from build123d import *

# Parameters (mm, degrees)
SKETCH_1_R               = 40
SKETCH_2_R               = 33.35
SKETCH_3_R               = 2.2
CUT_EXTRUDE_1_DEPTH      = 57.789083608
SKETCH_4_R               = 4
CUT_EXTRUDE_2_DEPTH      = 3
OTHER_START              = -5
OTHER_1_OUTLINE_R        = 4
OTHER_1_OUTLINE_R_2      = 2.9
OTHER_1_OUTLINE_R_3      = 11
OTHER_1_OUTLINE_R_4      = 9
OTHER_1_DEPTH            = 1.5
CUT_EXTRUDE_START        = 27
SKETCH_5_R               = 11.2
SKETCH_5_R_2             = 4.2
CUT_EXTRUDE_3_DEPTH      = 1.5
SKETCH_7_R               = 2.2
EXTRUDE_1_DEPTH          = 5
HOLE_WIZARD_4_4_4_4_1_D  = 4.4
CUT_EXTRUDE_4_DEPTH      = 91.740732016
CUT_EXTRUDE_4_DEPTH_BACK = 91.740732016


# Read off the part's stored shape, not the designer's step: 型腔1
with BuildPart() as part:
    # 草图1 → 放样2 section 0
    with BuildSketch(Plane.XY):
        Circle(SKETCH_1_R)
    # 草图2 → 放样2 section 1
    with BuildSketch(Plane.XY.offset(-5)):
        Circle(SKETCH_2_R)
    loft()

    # 草图3 → 切除-拉伸1 (cut, through all)
    with BuildSketch(Plane(origin=(0, 0, -5), x_dir=(-1, 0, 0), z_dir=(0, 0, -1))):
        with Locations((-25.11473671, -14.5)):
            Circle(SKETCH_3_R)
        with Locations((25.11473671, -14.5)):
            Circle(SKETCH_3_R)
        with Locations((0, 29)):
            Circle(SKETCH_3_R)
    extrude(amount=-CUT_EXTRUDE_1_DEPTH, mode=Mode.SUBTRACT)

    # 草图4 → 切除-拉伸2 (cut)
    with BuildSketch(Plane.XY):
        with Locations((0, 29)):
            Circle(SKETCH_4_R)
        with Locations((25.11473671, -14.5)):
            Circle(SKETCH_4_R)
        with Locations((-25.11473671, -14.5)):
            Circle(SKETCH_4_R)
    extrude(amount=-CUT_EXTRUDE_2_DEPTH, mode=Mode.SUBTRACT)

    # 型腔1 outline → 型腔1 (cut)
    # profile 1 of 2: a face of its own
    with BuildSketch(Plane.XY.offset(OTHER_START)):
        with Locations((-16.670989023, -9.625)):
            Circle(OTHER_1_OUTLINE_R)
        with Locations((-16.670989023, -9.625)):
            Circle(OTHER_1_OUTLINE_R_2, mode=Mode.SUBTRACT)
    # profile 2 of 2: a face of its own
    with BuildSketch(Plane.XY.offset(OTHER_START)):
        Circle(OTHER_1_OUTLINE_R_3)
        Circle(OTHER_1_OUTLINE_R_4, mode=Mode.SUBTRACT)
    extrude(amount=OTHER_1_DEPTH, mode=Mode.SUBTRACT)

    # 草图5 → 切除-拉伸3 (cut)
    with BuildSketch(Plane(origin=(52.090644265, -18.098750786, 23.5), x_dir=(0.9659258262890773, -0.2588190451024873, 0), z_dir=(0, 0, -1)).offset(CUT_EXTRUDE_START)):
        with Locations(Location((-55, -4, 0), (0, 0, 345))):
            Circle(SKETCH_5_R)
        with Locations(Location((-68.611805538, 9.611805538, 0), (0, 0, 345))):
            Circle(SKETCH_5_R_2)
    extrude(amount=CUT_EXTRUDE_3_DEPTH, mode=Mode.SUBTRACT)

    # 草图7 → 凸台-拉伸1 (add)
    # profile 1 of 5: a face of its own
    with BuildSketch(Plane.XY):
        with BuildLine():
            Line((56.314218304, 32.201068565), (22.765462134, 32.889720793))
            ThreePointArc((22.765462134, 32.889720793), (35.43034353, 18.565849222), (40, 0))
            ThreePointArc((40, 0), (39.957063165, -1.852863527), (39.828344838, -3.701749249))
            Line((39.828344838, -3.701749249), (60.865531412, 22.440746108))
            ThreePointArc((60.865531412, 22.440746108), (61.628929518, 28.738041798), (56.314218304, 32.201068565))
        make_face()
        with Locations((56.191082796, 26.202332228)):
            Circle(SKETCH_7_R, mode=Mode.SUBTRACT)
    # profile 2 of 5: a face of its own
    with BuildSketch(Plane.XY):
        with BuildLine():
            Line((-13.477261693, 37.661165904), (-46.06110803, 45.679035969))
            ThreePointArc((-46.06110803, 45.679035969), (-53.34269802, 41.195056807), (-48.745228802, 33.984585346))
            add(Edge.make_bspline(
                [(-48.745228802, 33.984585346), (-43.952768946, 31.311585993), (-37.935277565, 26.17758836), (-34.474104128, 20.286353653)],
                knots=[0, 0, 0, 0, 0.622020345, 0.622020345, 0.622020345, 0.622020345], degree=3))
            ThreePointArc((-34.474104128, 20.286353653), (-25.50106657, 30.81713166), (-13.477261693, 37.661165904))
        make_face()
        with Locations((-47.494755473, 39.852831801)):
            Circle(SKETCH_7_R, mode=Mode.SUBTRACT)
    # profile 3 of 5: a face of its own
    with BuildSketch(Plane.XY):
        with BuildLine():
            Line((4.379699915, 33.26712364), (-13.477261693, 37.661165904))
            ThreePointArc((-13.477261693, 37.661165904), (-25.50106657, 30.81713166), (-34.474104128, 20.286353653))
            add(Edge.make_bspline(
                [(-34.474104128, 20.286353653), (-33.715659981, 18.995412138), (-31.952819591, 15.314686764), (-31.439882273, 11.492206468), (-32.192854649, 8.708766247)],
                knots=[0.622020345, 0.622020345, 0.622020345, 0.622020345, 0.758323162, 1, 1, 1, 1], degree=3))
            ThreePointArc((-32.192854649, 8.708766247), (4.392652812, 33.059447988), (33.35, 0))
            ThreePointArc((33.35, 0), (31.454149072, -11.084178191), (25.982143558, -20.908149515))
            Line((25.982143558, -20.908149515), (39.828344838, -3.701749249))
            ThreePointArc((39.828344838, -3.701749249), (39.957063165, -1.852863527), (40, 0))
            ThreePointArc((40, 0), (35.43034353, 18.565849222), (22.765462134, 32.889720793))
            Line((22.765462134, 32.889720793), (4.379699915, 33.26712364))
        make_face()
    # profile 4 of 5: a face of its own
    with BuildSketch(Plane.XY):
        with BuildLine():
            ThreePointArc((10.561630861, -38.580460774), (-10.352761804, -38.637033052), (-28.436871018, -28.13084369))
            Line((-28.436871018, -28.13084369), (-21.933000593, -61.050335666))
            ThreePointArc((-21.933000593, -61.050335666), (-17.599695067, -65.682956188), (-11.530632138, -63.837641893))
            Line((-11.530632138, -63.837641893), (10.561630861, -38.580460774))
        make_face()
        with Locations((-16.046780796, -59.88740123)):
            Circle(SKETCH_7_R, mode=Mode.SUBTRACT)
    # profile 5 of 5: a face of its own
    with BuildSketch(Plane.XY):
        with BuildLine():
            Line((-32.717571704, -6.463977243), (-28.436871018, -28.13084369))
            ThreePointArc((-28.436871018, -28.13084369), (-10.352761804, -38.637033052), (10.561630861, -38.580460774))
            Line((10.561630861, -38.580460774), (25.102259624, -21.956754354))
            ThreePointArc((25.102259624, -21.956754354), (-8.631615154, -32.213626307), (-32.717571704, -6.463977243))
        make_face()
    extrude(amount=-EXTRUDE_1_DEPTH)

    # Ø4.4 (4.4) 直径孔1 (through all)
    with Locations(Plane(origin=(0, 0, -5), x_dir=(-1, 0, 0), z_dir=(0, 0, -1))):
        with Locations((10.352761804, -38.637033052), (-36.252311481, 16.90473047), (30.641777725, 25.711504387)):
            Hole(HOLE_WIZARD_4_4_4_4_1_D / 2)

    # 草图10 → 切除-拉伸4 (cut, two sides: drawn at the far end of the back side and taken through both)
    with BuildSketch(Plane(origin=(0, 0, -5), x_dir=(-1, 0, 0), z_dir=(0, 0, -1)).offset(-CUT_EXTRUDE_4_DEPTH_BACK)):
        Polygon((34.47410458, 20.28635588), (38.372841801, -16.056659606), (62.683016438, 23.101645648), align=None)
    extrude(amount=CUT_EXTRUDE_4_DEPTH + CUT_EXTRUDE_4_DEPTH_BACK, mode=Mode.SUBTRACT)


solid = part.part
Here's how the part is built. I have some questions about the finished solid (model axes, mm). A direction names the side the tool comes from. Round coordinates to 2 decimals unless told otherwise and drop trailing zeros. Write each loop counter-clockwise with the first axis right and the second up, starting at its lowest first coordinate (ties: lowest second). Pieces come first, ordered by that corner, then holes.
1. Suppose I cut it at A-A (x = 0). List the corners of the cut face in (y, z) for me.
2. Suppose I cut it at D-D (z = -1.65). State how many separate pieces and enclosed holes the cut face has, and give its area (3 significant figures).
3. Suppose I cut it at C-C (x = -16). List the corners of the cut face in (y, z) for me, and give its area (3 significant figures).
4. Will these pins go through, and if not, where does the flat tip stop? pin 1 Ø11 at (x, y) = (-16.67, -9.63) entering from -Z; pin 2 Ø4 at (x, y) = (0, 29) entering from -Z; pin 3 Ø2.5 at (x, y) = (-26.5, -13) entering from +Z; pin 4 Ø4 at (x, y) = (-18, -10) entering from -Z.
5. I need wall thicknesses on L1, parallel to X at y = 28, z = -2.45; L2, parallel to X at y = 1.5, z = -4.15; L3, parallel to X at y = 0, z = -4.3. Which ranges of each line are inside material? Lowest first, please.
6. If we mould it in two halves opening along Y, with no side actions, what happens to faces 1 (the conical face through (5.036, 36.385, -2.457)), 2 (the conical face through (27.9, -23.8, -2.5)), 3 (the flat face through (-36.21, 4.12, -1.02))? For each: released by +Y, released by -Y, zero draft, split by the parting line, or undercut.
7. Suppose I cut it at B-B (y = 0). List the corners of the cut face in (x, z) for me, and give its area (3 significant figures).
8. For faces 4 (the flat face through (-23, -16, -3)), 5 (the cylindrical face through (58.29, 26.86, -2.46)), 6 (the cylindrical face through (-14.73, -5.9, -4.24)), which set-ups out of +Z, -Z, +X, -X, +Y, -Y let a thin tool reach every point of the face, with its end or its side?
Answer sheet:
1. outline: (-50.66, -5) - (-11.2, -5) - (-11.2, -3.5) - (11.2, -3.5) - (11.2, -5) - (26.8, -5) - (26.8, -3) - (25, -3) - (25, 0) - (-50.66, 0) - close; (31.2, -5) - (34.34, -5) - (34.34, -4.25) - (40, 0) - (33, 0) - (33, -3) - (31.2, -3) - close
2. separate pieces: 1
2. enclosed holes: 9
2. area: 6,250 mm2
3. outline: (-65.89, -5) - (-62.09, -5) - (-62.09, 0) - (-65.89, 0) - close; (-57.69, -5) - (-13.77, -5) - (-13.77, -3.5) - (-5.48, -3.5) - (-5.48, -5) - (38.28, -5) - (38.28, 0) - (-57.69, 0) - close
3. area: 486 mm2
4. pin 1: stops at z = -5
4. pin 2: passes through
4. pin 3: stops at z = -3
4. pin 4: stops at z = -3.5
5. L1: x = -40.75 to -3.87, 3.87 to 54.92, 57.46 to 61.92
5. L2: x = -34.45 to -11.1, 11.1 to 44.01
5. L3: x = -34.28 to -11.2, 11.2 to 42.81
6. face 1: released by +Y
6. face 2: released by -Y
6. face 3: undercut
7. outline: (-36.65, -2.52) - (-33.35, -5) - (-11.2, -5) - (-11.2, -3.5) - (11.2, -3.5) - (11.2, -5) - (42.81, -5) - (42.81, 0) - (-36.65, 0) - close
7. area: 360 mm2
8. face 4: +Z
8. face 5: +Z, -Z
8. face 6: -Z
